Geometry check sheet. Reference: the model listing, model coordinates, mm. Coordinates: 2 decimals unless noted, no trailing zeros. Write each loop counter-clockwise with the first axis right and the second up, starting at its lowest first coordinate (ties: lowest second). Pieces come first, ordered by that corner, then holes. Notation, with made-up numbers: M -28,44.25 L -5,44.25 A10 cw -5,57.25 Z; hole C -15,2 d6. An arc over 180 degrees is marked long. Put each result on its own line as item: value. Start each with the question number.
1) Scan lines: line 1 along X through (y, z) = (-2.75, 15.5); line 2 along Y through (x, z) = (4.25, -109). Record each from-to range of solid material in increasing order.
2) Gauge pin test, flat ends, axial feed: pin 1 (1 mm diameter, centred on x = -2.5, y = -0.5, fed in from +Z); pin 2 (0.6 mm diameter, centred on x = -2.5, y = -1, fed in from -Z); pin 3 (6 mm diameter, centred on x = 8.5, z = 49, fed in from -Y). Record the tip position at first contact, or that the pin passes through.
3) Cross-section at B-B on x = -7.5. Record the cut outline in (y, z).
4) Cross-section at A-A on z = -25. Record the cut outline in (x, y).
5) Cross-section at C-C on y = -6.5. Record the cut outline in (x, z).
from build123d import *

# Parameters (mm, degrees)
RESSALTO_EXTRUS_O1_DEPTH = 182
CORTE_EXTRUS_O1_DEPTH    = 50
ESBO_O3_W                = 2.5
ESBO_O3_H                = 100
CORTE_EXTRUS_O2_DEPTH    = 185.202198684
CORTE_EXTRUS_O3_DEPTH    = 50


with BuildPart() as part:
    # Esboço1 → Ressalto-extrusão1 (new, symmetric)
    with BuildSketch(Plane.XY):
        Polygon((-12.7, 0), (12.7, 0), (12.7, -2), (1, -2), (1, -25.4), (-1, -25.4), (-1, -2), (-12.7, -2), align=None)
    extrude(amount=RESSALTO_EXTRUS_O1_DEPTH, both=True)

    # Esboço2 → Corte-extrusão1 (cut, symmetric)
    with BuildSketch(Plane(origin=(0, 0, 0), x_dir=(1, 0, 0), z_dir=(0, 1, 0))):
        Polygon((-1, 182), (12.7, 168.3), (12.7, 182), align=None)
        Polygon((-1, -182), (12.7, -168.3), (12.7, -182), align=None)
    extrude(amount=CORTE_EXTRUS_O1_DEPTH, both=True, mode=Mode.SUBTRACT)

    # Esboço3 → Corte-extrusão2 (cut, through all)
    with BuildSketch(Plane(origin=(0, 0, 0), x_dir=(1, 0, 0), z_dir=(0, 1, 0))):
        with Locations((-2.25, 70)):
            Rectangle(ESBO_O3_W, ESBO_O3_H)
        with Locations((-2.25, -70)):
            Rectangle(ESBO_O3_W, ESBO_O3_H)
    extrude(amount=-CORTE_EXTRUS_O2_DEPTH, mode=Mode.SUBTRACT)

    # Esboço4 → Corte-extrusão3 (cut, symmetric)
    with BuildSketch(Plane(origin=(0, 0, 0), x_dir=(1, 0, 0), z_dir=(0, 1, 0))):
        Polygon((-1, 182), (-12.7, 170.3), (-12.7, 182), align=None)
        Polygon((-1, -182), (-12.7, -170.3), (-12.7, -182), align=None)
    extrude(amount=CORTE_EXTRUS_O3_DEPTH, both=True, mode=Mode.SUBTRACT)


solid = part.part
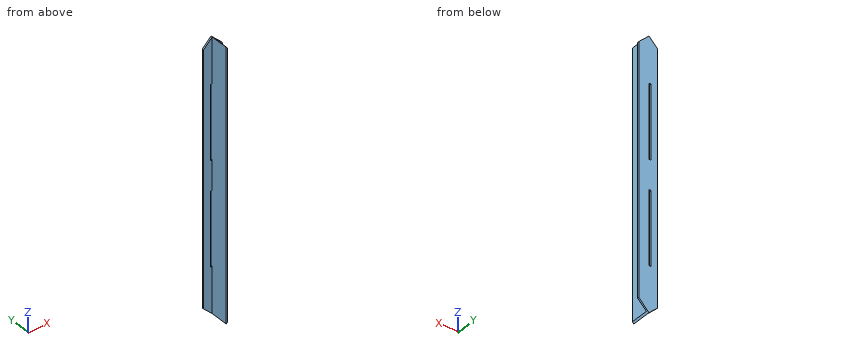
Answer key:
1. line 1: x = -1 to 1
1. line 2: y = -2 to 0
2. pin 1: stops at z = 181
2. pin 2: stops at z = -180.8
2. pin 3: stops at y = -2
3. outline: M -2,-175.5 L 0,-175.5 L 0,175.5 L -2,175.5 Z
4. outline: M -12.7,-2 L -3.5,-2 L -3.5,0 L -12.7,0 Z; M -1,-25.4 L 1,-25.4 L 1,-2 L 12.7,-2 L 12.7,0 L -1,0 Z
5. outline: M -1,-182 L 1,-180 L 1,180 L -1,182 Z
